Part model, mm, in its own coordinate system. A direction names the side the tool comes from. Round coordinates to 2 decimals unless told otherwise and drop trailing zeros. Loops run counter-clockwise (first coordinate to the right, second up) from the corner with the lowest first, then second, coordinate; pieces in that order, holes last. Notation, with made-up numbers: M 7.25,77.25 L 30.25,77.25 A20 cw 30.25,85.25 Z; hole C 44,30.25 d6. An arc over 180 degrees is marked long. Put each result on its own line as item: value. Start each with the question number.
1) Slice it at A-A on y = -233.5. Give the cut face in (x, z), then the cut area to 3 significant figures.
2) Slice it at C-C on x = -480.75. Give the cut face in (y, z), then the cut area to 3 significant figures.
3) Which spindle directions (+Z, -Z, +X, -X, +Y, -Y) get a long thin tool onto all of the face, cutting with end or side? Do faces 4 (the flat face through (-499.38, -242, 3)), 5 (the flat face through (-501.249, -230, 3)), 6 (the flat face through (-481.28, -230, 3)), 7 (the flat face through (-480, -244.906, 3)), 8 (the flat face through (-489.782, -233, 3)). Say none if no direction does.
4) Pull direction Y, two halves, no side cores. Call faces 1 (the flat face through (-492.03, -233, 3)), 2 (the flat face through (-483.18, -242, 3)), 3 (the flat face through (-504, -232.406, 3)): +Y half, -Y half, draft (parallel to the pull), parting line (faces both ways), or undercut.
5) Slice it at B-B on y = -242.25. Give the cut face in (x, z).
6) Probe line 1 along X through (y, z) = (-243.25, 2.65); line 2 along Y through (x, z) = (-490.5, 2); line 3 along X through (y, z) = (-230.25, 1.05). List the from-to ranges inside material, lowest first.
7) Slice it at D-D on y = -228.75. Give the cut face in (x, z).
```python
from build123d import *

# Parameters (mm, degrees)
BOSS_EXTRUDE1_DEPTH = 6


with BuildPart() as part:
    # Sketch1 → Boss-Extrude1 (new body)
    with BuildSketch(Plane.XY):
        Polygon((-477.021328122, -244.872375969), (-477.280147167, -244.906450143), (-482.180147167, -244.906450143), (-482.438966212, -244.872375969), (-482.680147167, -244.772475547), (-482.887253948, -244.613556924), (-483.046172571, -244.406450143), (-483.146072993, -244.165269188), (-483.180147167, -243.906450143), (-483.180147167, -239.906450143), (-499.380142171, -239.906450143), (-499.380142171, -243.906450143), (-499.414216344, -244.165269188), (-499.514116767, -244.406450143), (-499.67303539, -244.613556924), (-499.880142171, -244.772475547), (-500.121323126, -244.872375969), (-500.380142171, -244.906450143), (-505.248606329, -244.906450143), (-505.507425374, -244.872375969), (-505.748606329, -244.772475547), (-505.95571311, -244.613556924), (-506.114631732, -244.406450143), (-506.214532155, -244.165269188), (-506.248606329, -243.906450143), (-506.248606329, -232.406450143), (-501.248606329, -232.406450143), (-501.248606329, -228.406450143), (-501.214532155, -228.147631098), (-501.114631732, -227.906450143), (-500.95571311, -227.699343362), (-500.748606329, -227.540424739), (-500.507425374, -227.440524317), (-500.248606329, -227.406450143), (-482.280147167, -227.406450143), (-482.021328122, -227.440524317), (-481.780147167, -227.540424739), (-481.573040386, -227.699343362), (-481.414121763, -227.906450143), (-481.314221341, -228.147631098), (-481.280147167, -228.406450143), (-481.280147167, -232.406450143), (-476.280147167, -232.406450143), (-476.280147167, -243.906450143), (-476.314221341, -244.165269188), (-476.414121763, -244.406450143), (-476.573040386, -244.613556924), (-476.780147167, -244.772475547), align=None)
        Polygon((-492.029860545, -234.949153278), (-492.009763604, -235.045362548), (-491.949472778, -235.134152325), (-491.708309478, -235.2894734), (-491.346945625, -235.394834966), (-490.905956201, -235.429955488), (-490.464966776, -235.394834966), (-490.103602923, -235.2894734), (-489.862439623, -235.134152325), (-489.802148798, -235.045362548), (-489.782051856, -234.949153278), (-489.782051856, -231.602449772), (-489.802148798, -231.506259854), (-489.862439623, -231.417480498), (-490.103602923, -231.262153468), (-490.464966776, -231.156774038), (-490.905956201, -231.121647561), (-491.346945625, -231.156774038), (-491.708309478, -231.262153468), (-491.949472778, -231.417480498), (-492.009763604, -231.506259854), (-492.029860545, -231.602449772), align=None, mode=Mode.SUBTRACT)
    extrude(amount=BOSS_EXTRUDE1_DEPTH)


solid = part.part
```
Recorded:
1. outline: M -506.25,0 L -492.03,0 L -492.03,6 L -506.25,6 Z; M -489.78,0 L -476.28,0 L -476.28,6 L -489.78,6 Z
1. area: 166 mm2
2. outline: M -244.91,0 L -232.41,0 L -232.41,6 L -244.91,6 Z
2. area: 75.0 mm2
3. face 4: +Z, -Z, -Y
3. face 5: +Z, -Z, -X, +Y
3. face 6: +Z, -Z, +X, +Y
3. face 7: +Z, -Z, +X, -X, -Y
3. face 8: +Z, -Z
4. face 1: undercut
4. face 2: draft
4. face 3: +Y half
5. outline: M -506.25,0 L -499.38,0 L -499.38,6 L -506.25,6 Z; M -483.18,0 L -476.28,0 L -476.28,6 L -483.18,6 Z
6. line 1: x = -506.25 to -499.38, -483.18 to -476.28
6. line 2: y = -239.91 to -235.4, -231.15 to -227.41
6. line 3: x = -501.25 to -481.28
7. outline: M -501.25,0 L -481.28,0 L -481.28,6 L -501.25,6 Z
